Can you work these out from the model? Positions are in its coordinate system, mm. A direction names the side the tool comes from. Round coordinates to 2 decimals unless told otherwise and drop trailing zeros. Write each loop counter-clockwise with the first axis right and the second up, starting at its lowest first coordinate (ties: lowest second). Pieces come first, ordered by that corner, then holes. Notation, with made-up numbers: M 6.25,84 L 64.25,84 A25 ccw 64.25,116 Z; hole C -39,15.25 d5. An arc over 180 degrees is marked long. Answer as a JSON object with one key per item and string values. Group by question number.
1) Suppose I cut it at D-D, the plane y = 37. Write out the boundary of the cut face in (x, z), and give its area (3 significant figures).
2) Suppose I cut it at A-A, the plane x = -4.5. Write out the boundary of the cut face in (y, z), and give its area (3 significant figures).
3) Suppose I cut it at C-C, the plane x = 0. Write out the boundary of the cut face in (y, z).
4) If we mould it in two halves opening along X, with no side actions, what happens to faces 4 (the cylindrical face through (7.508, 60.963, -3.982)), 5 (the flat face through (0, 61.9, 0)), 6 (the cylindrical face through (-2.88, 9, -0.64))? For each: +X half, -X half, draft (parallel to the pull), parting line (faces both ways), or undercut.
5) Suppose I cut it at B-B, the plane z = 0. Write out the boundary of the cut face in (x, y), and give its area (3 significant figures).
6) Please list where these lines run through material, in increasing order: L1, parallel to Y at x = -3.75, z = -4.25; L2, parallel to X at y = 57.5, z = 0; L3, parallel to Y at x = 3.25, z = 7.5. Write a range as [from, to].
7) I'm going to push flat-ended pins straight in: pin 1 Ø6 at (y, z) = (41.5, 0) entering from +X; pin 2 Ø4 at (x, y) = (-2.5, 9) entering from +Z; pin 3 Ø8 at (y, z) = (36, -4.5) entering from -X. Where does each tip first touch, or does it pass through?
8) On a 3-axis mill with a long thin cutter (end or side, diameter ignored), from which of +Z, -Z, +X, -X, +Y, -Y can I reach the whole of each face in a straight line? I mean faces 1 (the flat face through (-2.1, 60, -2.4)), 2 (the cylindrical face through (1.802, 28.39, -5.723)), 3 (the cylindrical face through (-9.76, 60.94, -2.17)). Say none if no direction works.
from build123d import *

# Parameters (mm, degrees)
ESQUISSE1_R             = 2.95
BOSS_EXTRU_1_DEPTH      = 60
ESQUISSE2_R             = 10
BOSS_EXTRU_2_DEPTH      = 3
ESQUISSE3_R             = 1.2
ENL_V_MAT_EXTRU_1_DEPTH = 10
ESQUISSE4_R             = 10
ESQUISSE4_R_2           = 1.2
ENL_V_MAT_EXTRU_2_DEPTH = 1.1
ESQUISSE5_R             = 6
BOSS_EXTRU_3_DEPTH      = 20


with BuildPart() as part:
    # Esquisse1 → Boss.-Extru.1 (new body)
    with BuildSketch(Plane(origin=(0, 0, 0), x_dir=(1, 0, 0), z_dir=(0, 1, 0))):
        with Locations(Location((0, 0, 0), (0, 0, 270))):
            Circle(ESQUISSE1_R)
    extrude(amount=BOSS_EXTRU_1_DEPTH)

    # Esquisse2 → Boss.-Extru.2 (add)
    with BuildSketch(Plane(origin=(0, 60, 0), x_dir=(1, 0, 0), z_dir=(0, 1, 0))):
        with Locations(Location((0, 0, 0), (0, 0, 270))):
            Circle(ESQUISSE2_R)
    extrude(amount=BOSS_EXTRU_2_DEPTH)

    # Esquisse3 → Enlèv. mat.-Extru.1 (cut)
    with BuildSketch(Plane(origin=(0, 63, 0), x_dir=(1, 0, 0), z_dir=(0, 1, 0))):
        with BuildLine():
            ThreePointArc((-5.538612634, -3.945094433), (-7.212207999, -3.663885339), (-7.493417094, -5.337480704))
            Line((-7.493417094, -5.337480704), (-6.516014864, -4.641287568))
            Line((-6.516014864, -4.641287568), (-5.538612634, -3.945094433))
        make_face()
        with BuildLine():
            Line((-6.516014864, -4.641287568), (-7.493417094, -5.337480704))
            ThreePointArc((-7.493417094, -5.337480704), (-6.150558078, -5.784284216), (-5.316014864, -4.641287568))
            ThreePointArc((-5.316014864, -4.641287568), (-5.373018216, -4.275830783), (-5.538612634, -3.945094433))
            Line((-5.538612634, -3.945094433), (-6.516014864, -4.641287568))
        make_face()
        with BuildLine():
            ThreePointArc((-3.441287568, 6.516014864), (-4.091483859, 7.582652516), (-5.337480704, 7.493417094))
            Line((-5.337480704, 7.493417094), (-4.641287568, 6.516014864))
            Line((-4.641287568, 6.516014864), (-3.945094433, 5.538612634))
            ThreePointArc((-3.945094433, 5.538612634), (-3.574649916, 5.966211155), (-3.441287568, 6.516014864))
        make_face()
        with BuildLine():
            Line((-4.641287568, 6.516014864), (-5.337480704, 7.493417094))
            ThreePointArc((-5.337480704, 7.493417094), (-5.618689798, 5.819821729), (-3.945094433, 5.538612634))
            Line((-3.945094433, 5.538612634), (-4.641287568, 6.516014864))
        make_face()
        with BuildLine():
            ThreePointArc((3.945094433, -5.538612634), (3.663885339, -7.212207999), (5.337480704, -7.493417094))
            Line((5.337480704, -7.493417094), (4.641287568, -6.516014864))
            Line((4.641287568, -6.516014864), (3.945094433, -5.538612634))
        make_face()
        with BuildLine():
            Line((4.641287568, -6.516014864), (5.337480704, -7.493417094))
            ThreePointArc((5.337480704, -7.493417094), (5.707925221, -7.065818573), (5.841287568, -6.516014864))
            ThreePointArc((5.841287568, -6.516014864), (5.191091278, -5.449377212), (3.945094433, -5.538612634))
            Line((3.945094433, -5.538612634), (4.641287568, -6.516014864))
        make_face()
        with Locations(Location((6.495771182, 4.62686821, 0), (0, 0, 270))):
            Circle(ESQUISSE3_R)
    extrude(amount=-ENL_V_MAT_EXTRU_1_DEPTH, mode=Mode.SUBTRACT)

    # Esquisse4 → Enlèv. mat.-Extru.2 (cut)
    with BuildSketch(Plane(origin=(0, 63, 0), x_dir=(1, 0, 0), z_dir=(0, 1, 0))):
        with Locations(Location((0, 0, 0), (0, 0, 270))):
            Circle(ESQUISSE4_R)
        with Locations(Location((4.641287568, -6.516014864, 0), (0, 0, 270))):
            Circle(ESQUISSE4_R_2, mode=Mode.SUBTRACT)
        with Locations(Location((-6.516014864, -4.641287568, 0), (0, 0, 270))):
            Circle(ESQUISSE4_R_2, mode=Mode.SUBTRACT)
        with Locations(Location((6.495771182, 4.62686821, 0), (0, 0, 270))):
            Circle(ESQUISSE4_R_2, mode=Mode.SUBTRACT)
        with Locations(Location((-4.641287568, 6.516014864, 0), (0, 0, 270))):
            Circle(ESQUISSE4_R_2, mode=Mode.SUBTRACT)
    extrude(amount=-ENL_V_MAT_EXTRU_2_DEPTH, mode=Mode.SUBTRACT)

    # Esquisse5 → Boss.-Extru.3 (add)
    with BuildSketch(Plane(origin=(0, 38.25, 0), x_dir=(-1, 0, 0), z_dir=(0, -1, 0))):
        with Locations(Location((0, 0, 0), (0, 0, 90))):
            Circle(ESQUISSE5_R)
    extrude(amount=BOSS_EXTRU_3_DEPTH)


solid = part.part
Results:
{
 "1": {"outline": "C 0,0 d12", "area": "113 mm^2"},
 "2": {"outline": "M 18.25,-3.97 L 38.25,-3.97 L 38.25,3.97 L 18.25,3.97 Z; M 60,-8.93 L 61.9,-8.93 L 61.9,-7.71 L 60,-7.71 Z; M 60,-5.32 L 61.9,-5.32 L 61.9,8.93 L 60,8.93 Z", "area": "188 mm^2"},
 "3": {"outline": "M 0,-2.95 L 18.25,-2.95 L 18.25,-6 L 38.25,-6 L 38.25,-2.95 L 60,-2.95 L 60,-10 L 61.9,-10 L 61.9,10 L 60,10 L 60,2.95 L 38.25,2.95 L 38.25,6 L 18.25,6 L 18.25,2.95 L 0,2.95 Z"},
 "4": {"face 4": "undercut", "face 5": "draft", "face 6": "parting line"},
 "5": {"outline": "M -10,60 L -2.95,60 L -2.95,38.25 L -6,38.25 L -6,18.25 L -2.95,18.25 L -2.95,0 L 2.95,0 L 2.95,18.25 L 6,18.25 L 6,38.25 L 2.95,38.25 L 2.95,60 L 10,60 L 10,61.9 L -10,61.9 Z", "area": "514 mm^2"},
 "6": {"L1": "[18.25, 38.25], [60, 61.9]", "L2": "[-2.95, 2.95]", "L3": "[60, 61.9]"},
 "7": {"pin 1": "x = 2.95", "pin 2": "z = 2.91", "pin 3": "x = -5.98"},
 "8": {"face 1": "none", "face 2": "-Y", "face 3": "+Y, -Y"}
}
